```python
from build123d import *

# Parameters (mm, degrees)
SKETCH030_W  = 27
SKETCH030_H  = 22
PAD020_DEPTH = 2
SKETCH031_W  = 21
SKETCH031_H  = 19
PAD021_DEPTH = 3
SKETCH032_R  = 18.398369
PAD022_DEPTH = 4
SKETCH033_R  = 13
PAD023_DEPTH = 4
SKETCH034_W  = 22
SKETCH034_H  = 80
PAD024_DEPTH = 80
FILLET_R     = 5


with BuildPart() as part:
    # Sketch030 → Pad020 (new body)
    with BuildSketch(Plane.XY):
        with Locations((0, -1.5)):
            Rectangle(SKETCH030_W, SKETCH030_H)
    extrude(amount=PAD020_DEPTH)

    # Sketch031 (on Face6 of Pad020) → Pad021 (join)
    with BuildSketch(Plane.XY.offset(2)):
        Rectangle(SKETCH031_W, SKETCH031_H)
    extrude(amount=PAD021_DEPTH)

    # Sketch032 (on Face11 of Pad021) → Pad022 (join)
    with BuildSketch(Plane.XY.offset(5)):
        Circle(SKETCH032_R)
    extrude(amount=PAD022_DEPTH)

    # Sketch033 (on Face3 of Pad022) → Pad023 (join)
    with BuildSketch(Plane.XY.offset(9)):
        Circle(SKETCH033_R)
    extrude(amount=PAD023_DEPTH)

    # Sketch034 (on Face11 of Pad023) → Pad024 (join)
    with BuildSketch(Plane.XY.offset(13)):
        Rectangle(SKETCH034_W, SKETCH034_H)
    extrude(amount=PAD024_DEPTH)

    # Fillet
    fillet_edges = [part.edges().sort_by_distance(p)[0] for p in [
        (0, -40, 93),
        (0, 40, 93),
        (0, -40, 13),
        (0, 40, 13),
    ]]
    fillet(fillet_edges, radius=FILLET_R)


with BuildPart() as part_1:
    # Body013 placement: moved
    add(part.part.moved(Location((0, 100, 28))))


solid = part_1.part
```
Work out the finished part from the listing and answer in its coordinate system (mm). A direction names the side the tool comes from. Give positions to 0.01 mm unless a question says otherwise; leave off trailing zeros. Write each loop counter-clockwise with the first axis right and the second up, starting at its lowest first coordinate (ties: lowest second). Pieces come first, ordered by that corner, then holes.
(1) The part is cut by section A-A on x = 0. Write down the section's boundary in (y, z).
Final values:
outline: (60, 46) arc R5 ccw to (65, 41) - (87, 41) - (87, 37) - (81.6, 37) - (81.6, 33) - (90.5, 33) - (90.5, 30) - (87.5, 30) - (87.5, 28) - (109.5, 28) - (109.5, 33) - (118.4, 33) - (118.4, 37) - (113, 37) - (113, 41) - (135, 41) arc R5 ccw to (140, 46) - (140, 116) arc R5 ccw to (135, 121) - (65, 121) arc R5 ccw to (60, 116) - close
(2) The part is cut by section D-D on x = -5.5. Write down the section's boundary in (y, z).
Final values:
outline: (60, 46) arc R5 ccw to (65, 41) - (88.22, 41) - (88.22, 37) - (82.44, 37) - (82.44, 33) - (90.5, 33) - (90.5, 30) - (87.5, 30) - (87.5, 28) - (109.5, 28) - (109.5, 33) - (117.56, 33) - (117.56, 37) - (111.78, 37) - (111.78, 41) - (135, 41) arc R5 ccw to (140, 46) - (140, 116) arc R5 ccw to (135, 121) - (65, 121) arc R5 ccw to (60, 116) - close
(3) The mould has two halves that part along Z. Classify faces 1 (the flat face through (11, 99, 80)), 2 (the cylindrical face through (0, 139, 119)), 3 (the flat face through (10.5, 100, 31)): pulls with the +Z half, pulls with the -Z half, needs draft (parallel to the pull), parting line crosses it, or undercut.
Final values:
face 1: needs draft
face 2: pulls with the +Z half
face 3: undercut
(4) Which of the six approach directions +Z, -Z, +X, -X, +Y, -Y give full straight-line access (tool end or side, diameter ignored) to faces 4 (the flat face through (-11, 99, 80)), 5 (the flat face through (12, 100, 33)), 6 (the flat face through (0, 90.5, 31)), 7 (the flat face through (12, 100, 41))?
Final values:
face 4: +Z, -X, +Y, -Y
face 5: none
face 6: +X, -X, -Y
face 7: +Z, +X, +Y, -Y
(5) Straight lines are drawn through the part: line 1 (Z direction, x = -3, y = 89); line 2 (Z direction, x = 12.5, y = 103); line 3 (X direction, y = 67.5, z = 112). For each, find the intervals that lie inside material, in ascending order.
Final values:
line 1: z = 28 to 30, 33 to 121
line 2: z = 28 to 30, 33 to 41
line 3: x = -11 to 11
(6) Flat-ended cylindrical pins translate along their axes: pin 1 Ø17.5 at (x, y) = (1, 120.5) entering from -Z; pin 2 Ø0.9 at (y, z) = (97, 32) entering from +X; pin 3 Ø2 at (y, z) = (103.5, 29.5) entering from -X. Find the tip coordinate at first contact, or state that the pin passes through.
Final values:
pin 1: stops at z = 33
pin 2: stops at x = 10.5
pin 3: stops at x = -13.5
(7) The part is cut by section B-B on y = 100. Write down the section's boundary in (x, z).
Final values:
outline: (-18.4, 33) - (-10.5, 33) - (-10.5, 30) - (-13.5, 30) - (-13.5, 28) - (13.5, 28) - (13.5, 30) - (10.5, 30) - (10.5, 33) - (18.4, 33) - (18.4, 37) - (13, 37) - (13, 41) - (11, 41) - (11, 121) - (-11, 121) - (-11, 41) - (-13, 41) - (-13, 37) - (-18.4, 37) - close
(8) The part is cut by section C-C on z = 87. Write down the section's boundary in (x, y).
Final values:
outline: (-11, 60) - (11, 60) - (11, 140) - (-11, 140) - close
